Can you work these out from the model? Positions are in its coordinate system, mm. Round coordinates to 2 decimals unless told otherwise and drop trailing zeros. Loops run counter-clockwise (first coordinate to the right, second up) from the corner with the lowest first, then second, coordinate; pieces in that order, holes last. Notation, with made-up numbers: (16, 19.5) - (36, 19.5) arc R6 ccw to (36, 29.5) - close; hole circle Ø3 at (-20.75, -38). An arc over 180 degrees is marked (long way). Answer as CSV lines item,"result".
```python
from build123d import *

# Parameters (mm, degrees)
AUFSATZ_LINEAR_AUSTRAGEN1_DEPTH           = 120
AUFSATZ_LINEAR_AUSTRAGEN1_DEPTH_BACK      = 120
SKIZZE1_W                                 = 8
SKIZZE1_H                                 = 10
M5_GEWINDEBOHRUNG1_D                      = 4.2
F_4_2_4_2_DURCHMESSER_BOHRUNG1_AT_2_COUNT = 2
F_4_2_4_2_DURCHMESSER_BOHRUNG1_AT_2_PITCH = 70


with BuildPart() as part:
    # Skizze1 → Aufsatz-Linear austragen1 (new, two sides: drawn at the far end of the back side and taken through both)
    with BuildSketch(Plane.XY.offset(-AUFSATZ_LINEAR_AUSTRAGEN1_DEPTH_BACK)):
        Rectangle(SKIZZE1_W, SKIZZE1_H)
    extrude(amount=AUFSATZ_LINEAR_AUSTRAGEN1_DEPTH + AUFSATZ_LINEAR_AUSTRAGEN1_DEPTH_BACK)

    # M5 Gewindebohrung1 (through all)
    with Locations(Plane(origin=(0, 5, 0), x_dir=(1, 0, 0), z_dir=(0, 1, 0))):
        with Locations((0, -115), (0, -45)):
            m5_gewindebohrung1 = Hole(M5_GEWINDEBOHRUNG1_D / 2)

    # Skizze4 → Ø4.2 (4.2) Durchmesser Bohrung1 (revolve, cut)
    with BuildSketch(Plane(origin=(-4, 0, 105), x_dir=(0, 0, 1), z_dir=(0, 1, 0))):
        Polygon((0, 0), (0, 11.2618073), (2.1, 10), (2.1, 0), align=None)
    f_4_2_4_2_durchmesser_bohrung1 = revolve(axis=Axis((-10.35, 0, 105), (1, 0, 0)), mode=Mode.SUBTRACT)

    # Ø4.2 (4.2) Durchmesser Bohrung1 at 2: Ø4.2 (4.2) Durchmesser Bohrung1 ×2
    with Locations(*[(0, 0, -i * F_4_2_4_2_DURCHMESSER_BOHRUNG1_AT_2_PITCH) for i in range(1, F_4_2_4_2_DURCHMESSER_BOHRUNG1_AT_2_COUNT)]):
        add(f_4_2_4_2_durchmesser_bohrung1, mode=Mode.SUBTRACT)

    # Spiegeln1: M5 Gewindebohrung1, Ø4.2 (4.2) Durchmesser Bohrung1 across plane
    add(m5_gewindebohrung1.mirror(Plane.XY), mode=Mode.SUBTRACT)
    add(f_4_2_4_2_durchmesser_bohrung1.mirror(Plane.XY), mode=Mode.SUBTRACT)

    # Spiegeln1 copy 1 sketch → Spiegeln1 copy 1 (revolve, cut)
    with BuildSketch(Plane(origin=(-4, 0, -35), x_dir=(0, 0, -1), z_dir=(0, 1, 0))):
        Polygon((0, 0), (0, -11.2618073), (2.1, -10), (2.1, 0), align=None)
    revolve(axis=Axis((-10.35, 0, -35), (-1, 0, 0)), mode=Mode.SUBTRACT)


solid = part.part
```
Q1. We'd pull the mould along Z, two halves only. Please class faces 1 (the flat face through (0, -5, -2)), 2 (the flat face through (0, 0, 120)), 3 (the cylindrical face through (0.46, -0.07, -117.05)): pulls with the +Z half, pulls with the -Z half, needs draft (parallel to the pull), parting line crosses it, or undercut.
Checks:
face 1,"needs draft"
face 2,"pulls with the +Z half"
face 3,"undercut"
Q2. Imagine slicing it at B-B (x = 0). Count the separate pieces of the cut face and the enclosed holes in it, then the cut area to 3 significant figures.
Checks:
separate pieces,"5"
enclosed holes,"4"
area,"2,180 mm²"
Q3. I'm going to push a flat-ended pin straight in: pin 1 Ø4 at (x, z) = (0, -115) entering from +Y. Where does the tip first touch, or does it pass through?
Checks:
pin 1,"through"
Q4. Imagine slicing it at A-A (z = -35). Write out the boundary of the cut face in (x, y).
Checks:
outline,"(-4, -5) - (4, -5) - (4, -2.1) - (-4, -2.1) - close; (-4, 2.1) - (4, 2.1) - (4, 5) - (-4, 5) - close"
Q5. If I drill on line 1 along Z through (x, y) = (-1.25, -3); line 2 along X through (y, z) = (-1, 115); line 3 along Z through (x, y) = (3.25, -0.5), over which ranges is the centre line in solid material (lowest first)? Write a range as [from, to].
Checks:
line 1,"[-120, -116.69], [-113.31, -46.69], [-43.31, 43.31], [46.69, 113.31], [116.69, 120]"
line 2,"[-4, -2.1], [2.1, 4]"
line 3,"[-120, -107.04], [-102.96, -37.04], [-32.96, 32.96], [37.04, 102.96], [107.04, 120]"
